Autodesk Inventor part; units mm, degrees
ref_plane "YZ Plane" through (0, 0, 0) normal (1, 0, 0) x (0, 1, 0)
ref_plane "XZ Plane" through (0, 0, 0) normal (0, 1, 0) x (-1, 0, 0)
ref_plane "XY Plane" through (0, 0, 0) normal (0, 0, 1) x (1, 0, 0)
sketch "Sketch1" plane through (0, 0, 0) normal (0, 0, 1) x (1, 0, 0)
  line L0 (0, 0) -> (9.525, 0)
  line L1 (9.525, 0) -> (9.525, -95.25)
  line L2 (9.525, -95.25) -> (0, -95.25)
  line L3 (0, -95.25) -> (0, 0)
  dimension "d0" = 9.525
  dimension "d1" = 95.25
extrude "Extrusion1" add sketch "Sketch1" along normal blind 25.4
sketch "Sketch2" plane through (9.525, -95.25, 0) normal (1, 0, 0) x (0, 0, -1)
  line L0 (-25.4, 95.25) -> (-25.4, 0)
  line L1 (0, 95.25) -> (-25.4, 95.25)
  line L2 (-25.4, 95.25) -> (-25.4, 76.2)
  line L3 (-25.4, 76.2) -> (0, 76.2)
  line L4 (0, 76.2) -> (0, 95.25)
  dimension "d4" = 19.05
extrude "Extrusion2" add sketch "Sketch2" along normal blind 10.16
sketch "Sketch3" plane through (9.525, -95.25, 25.4) normal (1, 0, 0) x (0, 0, -1)
  line L0 (0, 0) -> (25.4, 0)
  line L1 (25.4, 0) -> (25.4, 9.525)
  line L2 (25.4, 9.525) -> (0, 9.525)
  line L3 (0, 9.525) -> (0, 0)
  point P0 (25.4, 95.25)
  dimension "d7" = 25.4
  dimension "d8" = 9.525
extrude "Extrusion3" add sketch "Sketch3" along normal blind 63.5
sketch "Sketch6" plane through (0, 0, 25.4) normal (0, 0, 1) x (1, 0, 0)
  point P0 (0, 0)
properties part number "door stop supreme"
The model under review builds one solid part; all positions refer to its coordinate system, in mm. A direction names the side the tool comes from. Give positions to 0.01 mm unless a question says otherwise; leave off trailing zeros. Loops run counter-clockwise (first coordinate to the right, second up) from the corner with the lowest first, then second, coordinate; pieces in that order, holes last. Notation, with made-up numbers: (-9.5, 47) -> (29.5, 47) arc R16 ccw to (29.5, 73) -> close; hole circle Ø8 at (54.5, -25). An arc over 180 degrees is marked (long way). Answer as a JSON object with one key per item and string values. Group by question number.
Q1. Take a section at D-D (x = 54). Write out the cut boundary in (y, z) (3 decimals).
Q2. Take a section at B-B (z = 17). Write out the cut boundary in (x, y) (3 decimals).
Q3. Tool access review of faces 1 (the flat face through (9.525, -52, 13)), 2 (the flat face through (36, -95.25, 13)), 3 (the flat face through (19.685, -9, 13)): name each direction out of +Z, -Z, +X, -X, +Y, -Y from which nothing blocks a thin tool from reaching the whole face with its end or side.
Q4. Wall thickness on line 1 along Y through (x, z) = (10.5, 3) (3 decimals); line 2 along X through (y, z) = (-59, 17.25) (3 decimals); line 3 along Y through (x, z) = (25, 5.75) (3 decimals): over which ranges is each line inside the solid? List them lowest first.
Q5. Insertion check: pin 1 (12 mm diameter, centred on y = -75.5, z = 10, fed in from -X); pin 2 (2 mm diameter, centred on y = -35, z = 5.5, fed in from +X) (3 decimals); pin 3 (5 mm diameter, centred on x = 53.5, z = 10.5, fed in from +Y) (3 decimals). Each pin has a flat end and moves straight along its axis. Give the tip position at first contact, or say it passes through.
Q6. Take a section at A-A (x = 12.5). Write out the cut boundary in (y, z) (3 decimals).
Q7. Draft analysis for pull direction Y (two halves, no side actions). For faces 4 (the flat face through (73.025, -90, 13)), 5 (the flat face through (10, 0, 13)), 6 (the flat face through (41, -85.725, 13)), state which applies: pulls with the +Y half, pulls with the -Y half, needs draft (parallel to the pull), parting line crosses it, or undercut.
Q8. Take a section at C-C (y = -25.5). Write out the cut boundary in (x, z) (3 decimals), plus the area to 3 significant figures.
Answer below:
{
 "1": {"outline": "(-95.25, 0) -> (-85.725, 0) -> (-85.725, 25.4) -> (-95.25, 25.4) -> close"},
 "2": {"outline": "(0, -95.25) -> (73.025, -95.25) -> (73.025, -85.725) -> (9.525, -85.725) -> (9.525, -19.05) -> (19.685, -19.05) -> (19.685, 0) -> (0, 0) -> close"},
 "3": {"face 1": "+Z, -Z, +X", "face 2": "+Z, -Z, +X, -X, -Y", "face 3": "+Z, -Z, +X, +Y"},
 "4": {"line 1": "y = -95.25 to -85.725, -19.05 to 0", "line 2": "x = 0 to 9.525", "line 3": "y = -95.25 to -85.725"},
 "5": {"pin 1": "stops at x = 0", "pin 2": "stops at x = 9.525", "pin 3": "stops at y = -85.725"},
 "6": {"outline": "(-95.25, 0) -> (-85.725, 0) -> (-85.725, 25.4) -> (-95.25, 25.4) -> close; (-19.05, 0) -> (0, 0) -> (0, 25.4) -> (-19.05, 25.4) -> close"},
 "7": {"face 4": "needs draft", "face 5": "pulls with the +Y half", "face 6": "undercut"},
 "8": {"outline": "(0, 0) -> (9.525, 0) -> (9.525, 25.4) -> (0, 25.4) -> close", "area": "242 mm2"}
}
